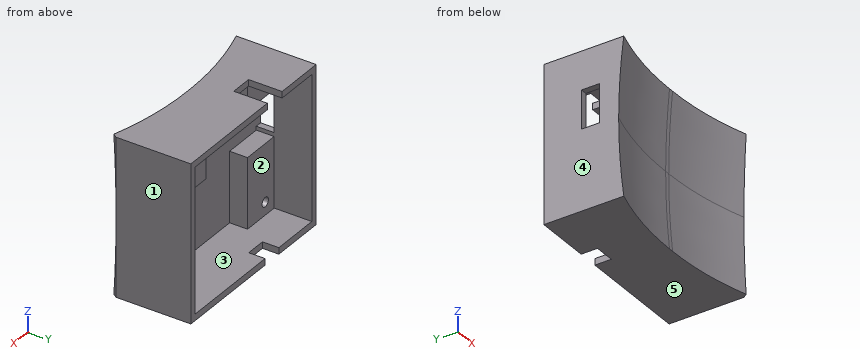
Autodesk Inventor part; units mm, degrees
ref_plane "Work Plane1" through (-33.95, 23.7, 2.5) normal (1, 0, 0) x (0, 0, -1)
ref_plane "YZ Plane" through (0, 0, 0) normal (1, 0, 0) x (0, 1, 0)
ref_plane "XZ Plane" through (0, 0, 0) normal (0, 1, 0) x (-1, 0, 0)
sketch "Sketch1" plane through (0, 0, 0) normal (0, 1, 0) x (-1, 0, 0)
  line L0 (0, 0) -> (67.9, 0)
  line L1 (67.9, 0) -> (67.9, -56.3)
  line L2 (67.9, -56.3) -> (0, -56.3)
  line L3 (0, -56.3) -> (0, 0)
  dimension "d4" = 67.9
  dimension "d5" = 56.3
extrude "Extrusion1" add sketch "Sketch1" along normal blind 2
sketch "Sketch4" plane through (0, 0, 0) normal (0, -1, 0) x (1, 0, 0)
  line L0 (2.5, 2.5) -> (-70.4, 2.5)
  line L1 (-70.4, 2.5) -> (-70.4, -58.8)
  line L2 (-70.4, -58.8) -> (2.5, -58.8)
  line L3 (2.5, -58.8) -> (2.5, 2.5)
  line L4 (0, -56.3) -> (0, 0)
  line L5 (0, 0) -> (-67.9, 0)
  line L6 (-67.9, -56.3) -> (0, -56.3)
  line L7 (-67.9, -56.3) -> (-67.9, 0)
  line L8 (0, 0) -> (-67.9, 0)
  line L9 (-67.9, 0) -> (-67.9, -56.3)
  line L10 (-67.9, -56.3) -> (0, -56.3)
  line L11 (0, -56.3) -> (0, 0)
  point P0 (-67.7799, -40.4535)
  point P1 (-67.7799, -17.6706)
  dimension "d35" = 2.5
  dimension "d36" = 2.5
  dimension "d37" = 2.5
  dimension "d38" = 2.5
extrude "Extrusion3" add sketch "Sketch4" against normal blind 23.7
sketch "Sketch5" plane through (2.5, 0, -58.8) normal (0, 0, -1) x (-1, 0, 0)
  line L0 (0, 0) -> (0, -5.5)
  line L1 (0, 0) -> (35.56, 0)
  line L2 (0, 0) -> (72.9, 0)
  arc A0 (35.56, 0) -> (0, -5.5) centre (35.56, -117.7058) ccw
  line L3 (72.9, 0) -> (0, 0)
  point P0 (2.5, 0)
  dimension "d41" = 5.5
  dimension "d42" = 35.56
extrude "Extrusion4" add sketch "Sketch5" against normal up to surface (61.3 mm away)
ref_plane "Work Plane1" through (-33.95, 23.7, 2.5) normal (1, 0, 0) x (0, 0, -1)
mirror "Mirror1" about plane through (-33.95, 23.7, 2.5) normal (1, 0, 0) of "Extrusion4"
sketch "Sketch11" plane through (0, 2, 0) normal (0, 1, 0) x (1, 0, 0)
  line L0 (-67.9, 0) -> (0, 0)
  line L1 (0, 0) -> (0, 56.3)
  line L2 (0, 56.3) -> (-67.9, 56.3)
  line L3 (-67.9, 56.3) -> (-67.9, 0)
  line L4 (-67.9, 0) -> (-52.5, 0)
  line L5 (-52.5, 0) -> (-52.5, 10.9)
  line L6 (-52.5, 10.9) -> (-67.9, 10.9)
  line L7 (-67.9, 10.9) -> (-67.9, 0)
  line L8 (-67.9, 56.3) -> (-52.4, 56.3)
  line L9 (-52.4, 56.3) -> (-52.4, 28.9)
  line L10 (-52.4, 28.9) -> (-67.9, 28.9)
  line L11 (-67.9, 28.9) -> (-67.9, 56.3)
  line L12 (0, 0) -> (-28.2, 0)
  line L13 (-28.2, 0) -> (-28.2, 24.4)
  line L14 (-28.2, 24.4) -> (0, 24.4)
  line L15 (0, 24.4) -> (0, 0)
  line L16 (0, 0) -> (0, 56.3)
  line L17 (0, 56.3) -> (-4, 56.3)
  line L18 (-4, 56.3) -> (-4, 29)
  line L19 (-4, 29) -> (0, 29)
  line L20 (0, 29) -> (0, 56.3)
  dimension "d89" = 15.4
  dimension "d90" = 10.9
  dimension "d91" = 15.5
  dimension "d92" = 27.4
  dimension "d93" = 28.2
  dimension "d94" = 24.4
  dimension "d95" = 4
  dimension "d96" = 27.3
extrude "Extrusion7" add sketch "Sketch11" along normal blind 7 contours L3 L6 L5 L0 | L13 L14 L1 L0 | L3 L2 L9 L10 | L19 L18 L2 L1
sketch "Sketch12" plane through (0, 9, 0) normal (0, 1, 0) x (1, 0, 0)
  line L0 (0, 0) -> (-67.9, 0)
  line L1 (-67.9, 0) -> (-67.9, 56.3)
  line L2 (-67.9, 56.3) -> (0, 56.3)
  line L3 (0, 56.3) -> (0, 0)
  point P0 (-62.6, 5.2)
  point P1 (-5.3, 5)
  point P2 (-62.7, 51.3)
  dimension "d99" = 5.2
  dimension "d100" = 5.3
  dimension "d101" = 5.2
  dimension "d102" = 5
  dimension "d103" = 5
  dimension "d104" = 5.3
hole "Hole6" at (-62.6, 9, -5.2) at (-5.3, 9, -5) at (-62.7, 9, -51.3) direction (0, -1, 0) diameter 3.7 depth 9
sketch "Sketch13" plane through (-70.4, 0, 2.5) normal (0, 0, 1) x (1, 0, 0)
  line L0 (17.9, 9) -> (2.5, 9)
  line L1 (70.4, 9) -> (42.2, 9)
  line L2 (19.8, 10.6) -> (28.4, 10.6)
  line L3 (28.4, 10.6) -> (28.4, 23.7)
  line L4 (28.4, 23.7) -> (19.8, 23.7)
  line L5 (19.8, 23.7) -> (19.8, 10.6)
  line L6 (0, 23.7) -> (72.9, 23.7)
  point P0 (70.4, 0)
  point P1 (2.5, 23.7)
  dimension "d112" = 1.6
  dimension "d113" = 17.3
  dimension "d114" = 8.6
extrude "Extrusion8" cut sketch "Sketch13" against normal up to surface (2.5 mm away)
sketch "Sketch14" plane through (-70.4, 0, -58.8) normal (-1, 0, 0) x (0, 0, 1)
  line L0 (5.65, 9) -> (9.35, 9)
  line L1 (29.9, 9) -> (2.5, 9)
  line L2 (29.9, 9) -> (2.5, 9)
  line L3 (58.8, 9) -> (47.9, 9)
  line L4 (51.75, 9) -> (55.45, 9)
  line L5 (58.8, 9) -> (47.9, 9)
  line L6 (58.8, 9) -> (47.9, 9)
  line L7 (31.4, 9) -> (46.4, 9)
  line L8 (46.4, 9) -> (46.4, 2)
  line L9 (46.4, 2) -> (31.4, 2)
  line L10 (31.4, 2) -> (31.4, 9)
  point P0 (58.8, 0)
  dimension "d118" = 12.4
  dimension "d119" = 15
  dimension "d120" = 7
extrude "Extrusion9" cut sketch "Sketch14" against normal up to surface (2.5 mm away)
sketch "Sketch15" plane through (2.5, 0, -58.8) normal (0, 0, -1) x (-1, 0, 0)
  line L0 (63.35, 9) -> (67.05, 9)
  line L1 (70.4, 9) -> (54.9, 9)
  line L2 (70.4, 9) -> (54.9, 9)
  line L3 (6.5, 9) -> (2.5, 9)
  line L4 (6.5, 9) -> (2.5, 9)
  line L5 (51.2, 23.7) -> (51.2, 17.3)
  line L6 (51.2, 17.3) -> (43.2, 17.3)
  line L7 (43.2, 17.3) -> (43.2, 23.7)
  line L8 (37.34, 0) -> (35.56, 0)
  line L9 (72.9, 23.7) -> (72.9, -5.5)
  line L10 (0, 23.7) -> (72.9, 23.7)
  line L11 (0, 23.7) -> (0, -5.5)
  arc A0 (35.56, 0) -> (0, -5.5) centre (35.56, -117.7058) ccw
  arc A1 (72.9, -5.5) -> (37.34, 0) centre (37.34, -117.7058) ccw
  line L12 (54.9, 2) -> (70.4, 2)
  line L13 (70.4, 2) -> (55, 2)
  line L14 (55, 2) -> (30.7, 2)
  line L15 (30.7, 2) -> (2.5, 2)
  line L16 (2.5, 2) -> (6.5, 2)
  line L17 (6.5, 2) -> (54.9, 2)
  line L18 (72.9, 2) -> (70.4, 2)
  line L19 (72.9, 2) -> (70.4, 2)
  point P0 (2.5, 0)
  dimension "d124" = 40.7
  dimension "d126" = 8.3
  dimension "d127" = 8
extrude "Extrusion10" cut sketch "Sketch15" against normal up to surface (2.5 mm away) contours L5 L6 L7 L10
sketch "Sketch16" plane through (-70.4, 23.7, -58.8) normal (-1, 0, 0) x (0, 0, 1)
  line L0 (0, -23.7) -> (61.3, -23.7)
  line L1 (0, -29.2) -> (0, -23.7)
  line L2 (61.3, 0) -> (61.3, -29.2)
  line L3 (0, -29.2) -> (61.3, -29.2)
  arc A0 (61.3, -31.2) -> (0, -31.2) centre (30.65, -265.0556) ccw
  line L4 (0, -29.2) -> (61.3, -29.2)
  line L5 (0, -31.2) -> (0, -29.2)
  line L6 (61.3, -29.2) -> (61.3, -31.2)
  point P0 (58.8, -23.7)
  point P1 (30.65, -26.2)
  dimension "d134" = 2
  dimension "d136" = 2
sketch3d "3D Sketch1"
  arc A0 (-70.4, -5.5, -58.8) -> (-34.84, 0, -58.8) centre (-34.84, -117.7058, -58.8) ccw
  line L0 (-34.84, 0, -58.8) -> (-33.06, 0, -58.8)
  arc A1 (-33.06, 0, -58.8) -> (2.5, -5.5, -58.8) centre (-33.06, -117.7058, -58.8) ccw
sweep "Sweep1" add profiles "Sketch16" path "3D Sketch1" contours L3 A0 L5 | L6 A0 L3
properties part number "Base"
Source: CAD feature listing. Evaluate the final solid. Frame: model axes, mm. Face numbers are marked on the shaded views. A direction names the side the tool comes from. Round coordinates to 2 decimals unless told otherwise and drop trailing zeros. Order: outer loops, then holes, each group sorted by start corner. A loop starts at its lowest first (then second) coordinate and runs counter-clockwise, first axis right, second up. Notation, with made-up numbers: (-15.5, -36) -> (8.5, -36) arc R23 ccw to (8.5, -21) -> close; hole circle Ø11 at (56.25, -3). An arc over 180 degrees is marked (long way). One line per item, written item: value. Start each with the question number.
Q1. Pin query (flat end, axial travel): pin 1 (1.2 mm diameter, centred on x = -45, z = 1, fed in from +Y); pin 2 (17 mm diameter, centred on x = -28, z = -30.5, fed in from +Y); pin 3 (1.2 mm diameter, centred on x = -44, z = -57, fed in from +Y). Return the tip coordinate at first contact, or that it passes through.
Q2. Draft query along Z for the marked faces 3, 4 and 5. Return one class per face: pulls with the +Z half, pulls with the -Z half, needs draft (parallel to the pull), parting line crosses it, or undercut.
Q3. Access query for the marked faces 1 and 2. Directions: +Z, -Z, +X, -X, +Y, -Y. A direction counts if a zero-diameter tool reaches every point of the face in a straight line with its end or side. Return the directions, or none.
Q4. Material intervals for probe 1 along X at (y, z) = (2.25, -5); probe 2 along Z at (x, y) = (-62.7, 2.75); probe 3 along Z at (x, y) = (-5.3, 2.5), sorted ascending.
Q5. Section query A-A (y = 4.5). Return the cut outline in (x, z), plus the area to 3 significant figures.
Findings below:
1. pin 1: y = 10.6
1. pin 2: y = 9
1. pin 3: y = 17.3
2. face 3: undercut
2. face 4: needs draft
2. face 5: pulls with the -Z half
3. face 1: +Z, -Z, +X, +Y, -Y
3. face 2: +Y
4. probe 1: -70.4 to -64.44, -60.76 to -52.5, -28.2 to -7.15, -3.45 to 2.5
4. probe 2: -58.8 to -53.15, -49.45 to -28.9, -10.9 to -7.05, -3.35 to 2.5
4. probe 3: -58.8 to -56.3, -24.4 to -6.85, -3.15 to 2.5
5. outline: (-70.4, -58.8) -> (2.5, -58.8) -> (2.5, 2.5) -> (-70.4, 2.5) -> (-70.4, -12.4) -> (-67.9, -12.4) -> (-67.9, -10.9) -> (-52.5, -10.9) -> (-52.5, 0) -> (-28.2, 0) -> (-28.2, -24.4) -> (0, -24.4) -> (0, -29) -> (-4, -29) -> (-4, -56.3) -> (-52.4, -56.3) -> (-52.4, -28.9) -> (-67.9, -28.9) -> (-67.9, -27.4) -> (-70.4, -27.4) -> close; hole circle Ø3.7 at (-62.7, -51.3); hole circle Ø3.7 at (-62.6, -5.2); hole circle Ø3.7 at (-5.3, -5)
5. area: 1,970 mm²
